Geometry check sheet. Reference: drawing and pictorial views, mm from the part's lowest x, y, z. A direction names the side the tool comes from. Give positions to 0.01 mm unless a question says otherwise; leave off trailing zeros. Write each loop counter-clockwise with the first axis right and the second up, starting at its lowest first coordinate (ties: lowest second). Pieces come first, ordered by that corner, then holes. Notation, with made-up numbers: (-22, -19) - (25, -19) arc R25 cw to (25, 3) - close; hole circle Ø1 at (74, 11). An arc over 180 degrees is marked (long way). Write item = value, one per line. Start each with the question number.
(1) Draft check along X on the marked faces 1, 2 and 3. Enter one of: pulls with the +X half, pulls with the -X half, needs draft (parallel to the pull), parting line crosses it, or undercut.
(2) Access from +Z, -Z, +X, -X, +Y, -Y to the whole of each face (thin tool, end or side, straight path). Record for the marked faces 4 and 5.
(3) Section check D-D, the plane x = 27. Enter the section's corners in (y, z).
(4) Depth check by flat-ended pin: pin 1 Ø5.5 at (x, z) = (6.35, 6.35) entering from -Y; pin 2 Ø2.5 at (x, y) = (26, 5) entering from +Z; pin 3 Ø0.6 at (x, y) = (7.5, 4) entering from -Z. Enter the tip coordinate at first touch or a pass-through.
(5) Thickness scan on L1, parallel to Z at x = 6.35, y = 7.4 (1 decimal); L2, parallel to Y at x = 9, z = 8. Record the ranges inside material, lowest first.
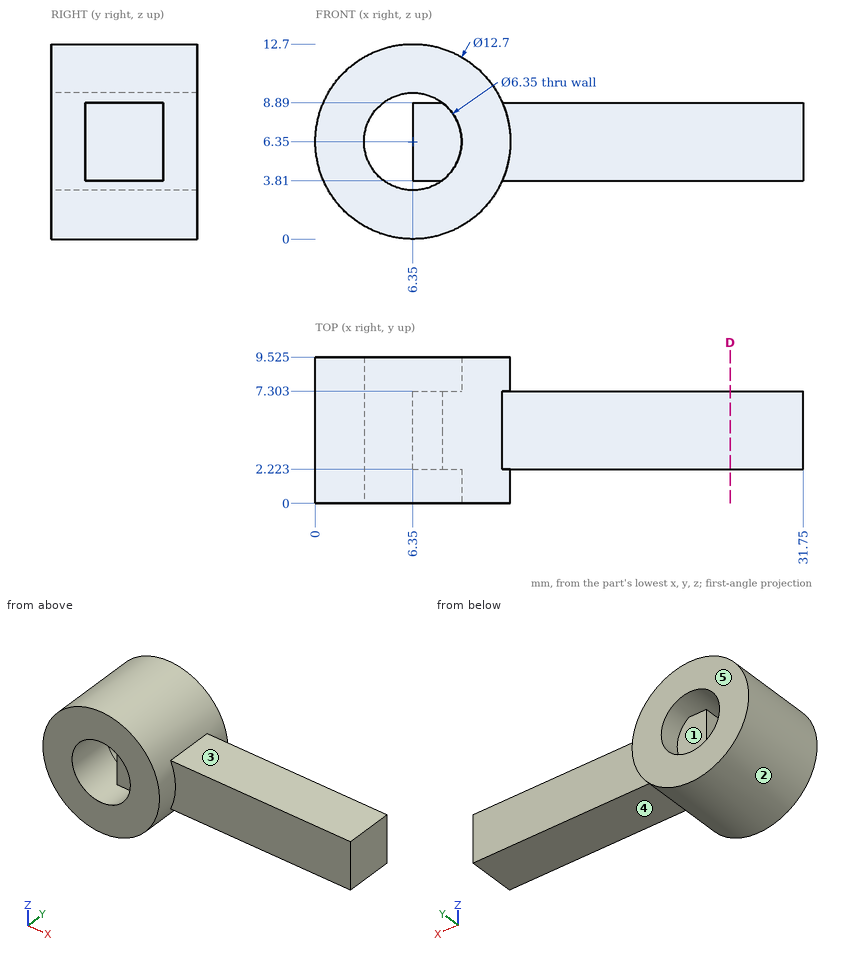
Model answer:
q1.face_1 = undercut
q1.face_2 = parting line crosses it
q1.face_3 = needs draft
q2.face_4 = -Z, +X, +Y, -Y
q2.face_5 = +Z, -Z, +X, -X, +Y
q3.outline = (2.22, 3.81) - (7.3, 3.81) - (7.3, 8.89) - (2.22, 8.89) - close
q4.pin_1 = 2.22
q4.pin_2 = 8.89
q4.pin_3 = 0.06
q5.L1 = 0 to 3.2, 9.5 to 12.7
q5.L2 = 2.22 to 7.3
